Geometry check sheet. Reference: the model listing, model coordinates, mm. A direction names the side the tool comes from. Round coordinates to 2 decimals unless told otherwise and drop trailing zeros. Write each loop counter-clockwise with the first axis right and the second up, starting at its lowest first coordinate (ties: lowest second). Pieces come first, ordered by that corner, then holes. Notation, with made-up numbers: M 53.25,21 L 62.25,21 A14 ccw 62.25,35 Z; hole C 75,21 d3. An arc over 180 degrees is marked long. Put each result on its own line as item: value. Start each with the question number.
(1) Tool access check on faces 1 (the flat face through (5, 0, 35.992)), 2 (the flat face through (-381, 11, 0)). Record the directions out of +Z, -Z, +X, -X, +Y, -Y that give a thin tool (end or side, any length) a straight path to the whole face; none if there is none.
(2) Section check D-D on z = -28. Record the cut outline in (x, y).
(3) Section check C-C on x = 0. Record the cut outline in (y, z), then the cut area to 3 significant figures.
(4) Mould release check, pull along X, two halves, no side actions. Record for faces 3 (the flat face through (5, -10.592, -17)), 4 (the cylindrical face through (-14.274, 11.631, 0.628)), 5 (the flat face through (381, 11, 0)): pulls with the +X half, pulls with the -X half, needs draft (parallel to the pull), parting line crosses it, or undercut.
(5) Material ranges on probe 1 along Y at (x, z) = (-176.5, -35); probe 2 along Z at (x, y) = (-111.5, -6.75); probe 3 along Z at (x, y) = (0, 12.1), recorded low to high.
(6) Section check A-A on y = -6.5. Record the cut outline in (x, z), then the cut area to 3 significant figures.
(7) Section check B-B on z = 0. Record the cut outline in (x, y), then the cut area to 3 significant figures.
from build123d import *

# Parameters (mm, degrees)
F0_W     = 25.4
F0_H     = 76.2
F0_W_2   = 21.1836
F0_H_2   = 71.9836
F1_DEPTH = 381
F2_R     = 14.2875
F3_DEPTH = 25.401


with BuildPart() as f1:
    # F0 (on Right) → F1 (new body, symmetric)
    with BuildSketch(Plane.YZ):
        Rectangle(F0_W, F0_H)
        Rectangle(F0_W_2, F0_H_2, mode=Mode.SUBTRACT)
    extrude(amount=F1_DEPTH, both=True)

    # F2 (on face) → F3 (cut, through all)
    with BuildSketch(Plane.XZ.offset(12.7)):
        Circle(F2_R)
    extrude(amount=-F3_DEPTH, mode=Mode.SUBTRACT)


solid = f1.part
Answers follow:
1. face 1: +X, -X
1. face 2: +Z, -Z, -X, +Y, -Y
2. outline: M -381,-12.7 L 381,-12.7 L 381,-10.59 L -381,-10.59 Z; M -381,10.59 L 381,10.59 L 381,12.7 L -381,12.7 Z
3. outline: M -12.7,-38.1 L 12.7,-38.1 L 12.7,-14.29 L 10.59,-14.29 L 10.59,-35.99 L -10.59,-35.99 L -10.59,-14.29 L -12.7,-14.29 Z; M -12.7,14.29 L -10.59,14.29 L -10.59,35.99 L 10.59,35.99 L 10.59,14.29 L 12.7,14.29 L 12.7,38.1 L -12.7,38.1 Z
3. area: 290 mm^2
4. face 3: needs draft
4. face 4: undercut
4. face 5: pulls with the +X half
5. probe 1: y = -12.7 to -10.59, 10.59 to 12.7
5. probe 2: z = -38.1 to -35.99, 35.99 to 38.1
5. probe 3: z = -38.1 to -14.29, 14.29 to 38.1
6. outline: M -381,-38.1 L 381,-38.1 L 381,-35.99 L -381,-35.99 Z; M -381,35.99 L 381,35.99 L 381,38.1 L -381,38.1 Z
6. area: 3,210 mm^2
7. outline: M -381,-12.7 L -14.29,-12.7 L -14.29,-10.59 L -381,-10.59 Z; M -381,10.59 L -14.29,10.59 L -14.29,12.7 L -381,12.7 Z; M 14.29,-12.7 L 381,-12.7 L 381,-10.59 L 14.29,-10.59 Z; M 14.29,10.59 L 381,10.59 L 381,12.7 L 14.29,12.7 Z
7. area: 3,090 mm^2
